The listing builds one solid part. Answer for the finished solid, in the listing's coordinates (mm). Coordinates: 2 decimals unless noted, no trailing zeros. Write each loop counter-clockwise with the first axis right and the second up, starting at its lowest first coordinate (ties: lowest second). Pieces come first, ordered by that corner, then holes. Notation, with made-up numbers: M 13,17 L 35,17 A17 cw 35,28 Z; hole C 61,40.25 d2. An arc over 180 degrees is marked long. Answer as a JSON object with one key per item and string values. Group by question number.
from build123d import *

# Parameters (mm, degrees)
F0_R     = 0.75
F1_DEPTH = 20
F2_R     = 0.6
F3_DEPTH = 3
F4_R     = 0.33
F5_DEPTH = 7
F6_R     = 0.235
F7_DEPTH = 7
F8_R     = 0.435
F9_DEPTH = 3


with BuildPart() as f1:
    # F0 (on Front) → F1 (new body)
    with BuildSketch(Plane.XZ):
        Circle(F0_R)
    extrude(amount=F1_DEPTH)

    # F2 (on face) → F3 (cut)
    with BuildSketch(Plane.XZ.offset(20)):
        Circle(F2_R)
    extrude(amount=-F3_DEPTH, mode=Mode.SUBTRACT)

    # F4 (on face) → F5 (cut)
    with BuildSketch(Plane.XZ.offset(17)):
        Circle(F4_R)
    extrude(amount=-F5_DEPTH, mode=Mode.SUBTRACT)

    # F6 (on face) + F4 (on face) → F7 (cut)
    with BuildSketch(Plane.XZ.offset(10)):
        Circle(F6_R)
    with BuildSketch(Plane.XZ.offset(17)):
        Circle(F4_R)
    extrude(amount=-F7_DEPTH, mode=Mode.SUBTRACT)

    # F8 (on face) → F9 (cut)
    with BuildSketch(Plane(origin=(0, 0, 0), x_dir=(-1, 0, 0), z_dir=(0, 1, 0))):
        Circle(F8_R)
    extrude(amount=-F9_DEPTH, mode=Mode.SUBTRACT)


solid = f1.part
Item 1: A cutting plane is placed at C-C, the plane y = -17.5. Write down the section's boundary in (x, z).
Item 2: A flat-ended cylindrical pin translates along its axis: pin 1 Ø0.6 at (x, z) = (0, 0) entering from -Y. Find the tip coordinate at first contact, or state that the pin passes through.
Item 3: A cutting plane is placed at D-D, the plane y = -11.5. Write down the section's boundary in (x, z).
Item 4: Consider L1, parallel to Z at x = 0, y = -7.75 (3 decimals); L2, parallel to Z at x = 0, y = -14.5; L3, parallel to Y at x = -0.2, z = -0.45. Determine where each line is inside the solid, lowest interval first. Write a range as from..to.
Item 5: For a pull along X with two mould halves and no side action, classify faces 1 (the face through (-0.75, -9.86, 0.03)), 2 (the face through (0.094, -1.479, -0.425)) as +X half, -X half, draft (parallel to the pull), parting line (faces both ways), or undercut.
Item 6: A cutting plane is placed at B-B, the plane z = 0. Write down the section's boundary in (x, y) (3 decimals), and give its area (3 significant figures).
Item 7: A cutting plane is placed at A-A, the plane x = 0. Write down the section's boundary in (y, z) (3 decimals), and give its area (3 significant figures).
Answer:
{
 "1": {"outline": "C 0,0 d1.5; hole C 0,0 d1.2"},
 "2": {"pin 1": "y = -10"},
 "3": {"outline": "C 0,0 d1.5; hole C 0,0 d0.66"},
 "4": {"L1": "-0.75..-0.235, 0.235..0.75", "L2": "-0.75..-0.33, 0.33..0.75", "L3": "-17..0"},
 "5": {"face 1": "parting line", "face 2": "undercut"},
 "6": {"outline": "M -0.75,-20 L -0.6,-20 L -0.6,-17 L -0.33,-17 L -0.33,-10 L -0.235,-10 L -0.235,-3 L -0.435,-3 L -0.435,0 L -0.75,0 Z; M 0.235,-10 L 0.33,-10 L 0.33,-17 L 0.6,-17 L 0.6,-20 L 0.75,-20 L 0.75,0 L 0.435,0 L 0.435,-3 L 0.235,-3 Z", "area": "15.9 mm2"},
 "7": {"outline": "M -20,-0.75 L 0,-0.75 L 0,-0.435 L -3,-0.435 L -3,-0.235 L -10,-0.235 L -10,-0.33 L -17,-0.33 L -17,-0.6 L -20,-0.6 Z; M -20,0.6 L -17,0.6 L -17,0.33 L -10,0.33 L -10,0.235 L -3,0.235 L -3,0.435 L 0,0.435 L 0,0.75 L -20,0.75 Z", "area": "15.9 mm2"}
}
